Verification items for this drawing (mm, ordinates from the low corner). Coordinates: 2 decimals unless noted, no trailing zeros. Order: outer loops, then holes, each group sorted by start corner. A loop starts at its lowest first (then second) coordinate and runs counter-clockwise, first axis right, second up. Notation, with made-up numbers: M 22,85 L 65,85 A28 cw 65,115 Z; hole C 85.25,2.5 d8. An arc over 180 degrees is marked long. Return JSON: item names as keys, results as strings. Group by question number.
1. Mould release check, pull along X, two halves, no side actions. Record for the marked faces 1, 2 and 3: +X half, -X half, draft (parallel to the pull), parting line (faces both ways), or undercut.
2. Section check A-A, the plane y = 24.5. Record the cut outline in (x, z), plus the area to 3 significant figures.
3. Section check C-C, the plane y = 38.5. Record the cut outline in (x, z).
4. Material ranges on line 1 along Z through (x, y) = (65, 10); line 2 along Y through (x, z) = (69.5, 25.5); line 3 along Z through (x, y) = (69, 18), recorded low to high.
5. Section check B-B, the plane x = 113.5. Record the cut outline in (y, z) (1 decimal), plus the area to 3 significant figures.
6. Gauge pin test, flat ends, axial feed: pin 1 (10 mm diameter, centred on x = 96.5, z = 22.5, fed in from -Y); pin 2 (21 mm diameter, centred on x = 65, z = 65, fed in from -Y); pin 3 (1.5 mm diameter, centred on x = 70.5, y = 34.5, fed in from +Z). Record the tip position at first contact, or that the pin passes through.
7. Section check D-D, the plane z = 112. Record the cut outline in (x, y).
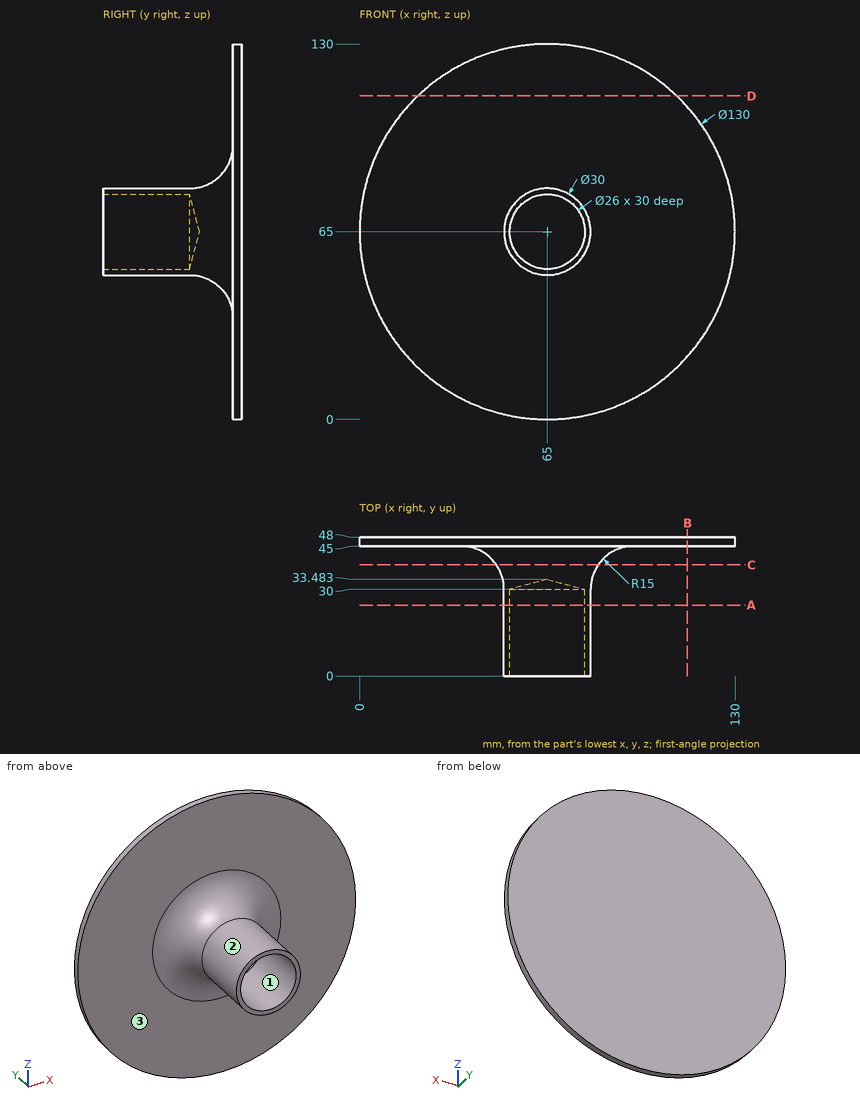
Answers follow:
{
 "1": {"face 1": "undercut", "face 2": "parting line", "face 3": "draft"},
 "2": {"outline": "C 65,65 d30; hole C 65,65 d26", "area": "176 mm^2"},
 "3": {"outline": "C 65,65 d35.28"},
 "4": {"line 1": "50 to 52, 78 to 80", "line 2": "45 to 48", "line 3": "50.54 to 52.63, 77.37 to 79.46"},
 "5": {"outline": "M 45,21.7 L 48,21.7 L 48,108.3 L 45,108.3 Z", "area": "260 mm^2"},
 "6": {"pin 1": "y = 45", "pin 2": "y = 30.67", "pin 3": "z = 80.07"},
 "7": {"outline": "M 20.1,45 L 109.9,45 L 109.9,48 L 20.1,48 Z"}
}
